Design review of the part built by this model. Coordinates are the model's own, in mm. Face numbers are marked on the shaded views. Coordinates: 2 decimals unless noted, no trailing zeros. Write each loop counter-clockwise with the first axis right and the second up, starting at its lowest first coordinate (ties: lowest second). Pieces come first, ordered by that corner, then holes.
Q1. The part is to be moulded in two halves that separate along X. For the marked faces 1, 2, 3 and 4, say which applies: +X half, -X half, draft (parallel to the pull), parting line (faces both ways), or undercut.
Q2. Add section A-A, the plane z = -25.5. Give the boundary of the cut face in (x, y), plus the area to 3 significant figures.
Q3. Clearance check with a flat-ended pin moving along its axis: pin 1 Ø11.5 at (x, z) = (40, -25.5) entering from +Y. State where the tip first meets the part, or that it passes through.
Q4. Add section C-C, the plane y = 2.25. Give the boundary of the cut face in (x, z), plus the area to 3 significant figures.
Q5. To check wall thickness, follow probe 1 along X at (y, z) = (10.5, -25.5); probe 2 along Z at (x, y) = (42.5, 9.75); probe 3 along X at (y, z) = (5.25, -18). State the ranges of each line that lie inside material, in increasing order.
Q6. Add section B-B, the plane x = 40. Give the boundary of the cut face in (y, z).
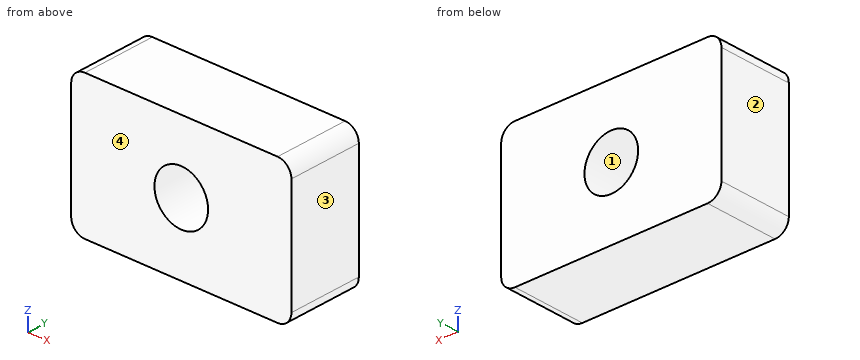
from build123d import *

# Parameters (mm, degrees)
CROQUIS1_W              = 80
CROQUIS1_H              = 51
SALIENTE_EXTRUIR1_DEPTH = 27
CROQUIS2_R              = 9.75
CORTAR_EXTRUIR1_DEPTH   = 27
REDONDEO1_R             = 5


with BuildPart() as part:
    # Croquis1 → Saliente-Extruir1 (new body)
    with BuildSketch(Plane(origin=(0, 0, 0), x_dir=(1, 0, 0), z_dir=(0, 1, 0))):
        with Locations((40, 25.5)):
            Rectangle(CROQUIS1_W, CROQUIS1_H)
    extrude(amount=SALIENTE_EXTRUIR1_DEPTH)

    # Croquis2 → Cortar-Extruir1 (cut)
    with BuildSketch(Plane(origin=(0, 27, 0), x_dir=(1, 0, 0), z_dir=(0, 1, 0))):
        with Locations(Location((40, 25.5, 0), (0, 0, 270))):
            Circle(CROQUIS2_R)
    extrude(amount=-CORTAR_EXTRUIR1_DEPTH, mode=Mode.SUBTRACT)

    # Redondeo1
    redondeo1_edges = [part.edges().sort_by_distance(p)[0] for p in [
        (0, 13.5, -51),
        (80, 13.5, -51),
        (80, 13.5, 0),
        (0, 13.5, 0),
    ]]
    fillet(redondeo1_edges, radius=REDONDEO1_R)


solid = part.part
Here are the results:
1. face 1: undercut
1. face 2: -X half
1. face 3: +X half
1. face 4: draft
2. outline: (0, 0) - (30.25, 0) - (30.25, 27) - (0, 27) - close; (49.75, 0) - (80, 0) - (80, 27) - (49.75, 27) - close
2. area: 1,630 mm2
3. pin 1: passes through
4. outline: (0, -46) arc R5 ccw to (5, -51) - (75, -51) arc R5 ccw to (80, -46) - (80, -5) arc R5 ccw to (75, 0) - (5, 0) arc R5 ccw to (0, -5) - close; hole circle Ø19.5 at (40, -25.5)
4. area: 3,760 mm2
5. probe 1: x = 0 to 30.25, 49.75 to 80
5. probe 2: z = -51 to -34.92, -16.08 to 0
5. probe 3: x = 0 to 33.77, 46.23 to 80
6. outline: (0, -51) - (27, -51) - (27, -35.25) - (0, -35.25) - close; (0, -15.75) - (27, -15.75) - (27, 0) - (0, 0) - close
